Check sheet for the modelled part. Datum: model origin and axes. Units: mm. Face numbers are marked on the shaded views. A direction names the side the tool comes from. Give positions to 0.01 mm unless a question says otherwise; leave off trailing zeros. Order: outer loops, then holes, each group sorted by start corner. A loop starts at its lowest first (then second) coordinate and runs counter-clockwise, first axis right, second up.
from build123d import *

# Parameters (mm, degrees)
DODANIE_WYCI_GNI_CIE1_DEPTH  = 20
ZAAWANSOWANYOTW_R1_START     = -11.5
ZAAWANSOWANYOTW_R1_OUTLINE_R = 5.5
ZAAWANSOWANYOTW_R1_DEPTH     = 23


# Read off the part's stored shape, not the designer's step: ZaawansowanyOtwór1
with BuildPart() as part:
    # Szkic1 → Dodanie-wyciągnięcie1 (new body)
    with BuildSketch(Plane(origin=(0, 0, 0), x_dir=(1, 0, 0), z_dir=(0, 1, 0))):
        with BuildLine():
            Line((12.109500403, 11.5), (39.7, 11.5))
            ThreePointArc((39.7, 11.5), (41.114213562, 10.914213562), (41.7, 9.5))
            Line((41.7, 9.5), (41.7, 4.5))
            ThreePointArc((41.7, 4.5), (41.114213562, 3.085786438), (39.7, 2.5))
            Line((39.7, 2.5), (13.774977314, 2.5))
            Line((13.774977314, 2.5), (12.939860896, 2.5))
            ThreePointArc((12.939860896, 2.5), (11.780953784, 2.869989477), (11.050830108, 3.843065693))
            ThreePointArc((11.050830108, 3.843065693), (-11.7, 0), (11.050830108, -3.843065693))
            ThreePointArc((11.050830108, -3.843065693), (11.780953784, -2.869989477), (12.939860896, -2.5))
            Line((12.939860896, -2.5), (13.774977314, -2.5))
            Line((13.774977314, -2.5), (39.7, -2.5))
            ThreePointArc((39.7, -2.5), (41.114213562, -3.085786438), (41.7, -4.5))
            Line((41.7, -4.5), (41.7, -9.5))
            ThreePointArc((41.7, -9.5), (41.114213562, -10.914213562), (39.7, -11.5))
            Line((39.7, -11.5), (12.109500403, -11.5))
            ThreePointArc((12.109500403, -11.5), (-16.7, 0), (12.109500403, 11.5))
        make_face()
    extrude(amount=DODANIE_WYCI_GNI_CIE1_DEPTH)

    # ZaawansowanyOtwór1 outline → ZaawansowanyOtwór1 (cut)
    with BuildSketch(Plane.XY.offset(ZAAWANSOWANYOTW_R1_START)):
        with Locations((31.7, 10)):
            Circle(ZAAWANSOWANYOTW_R1_OUTLINE_R)
    extrude(amount=ZAAWANSOWANYOTW_R1_DEPTH, mode=Mode.SUBTRACT)


solid = part.part
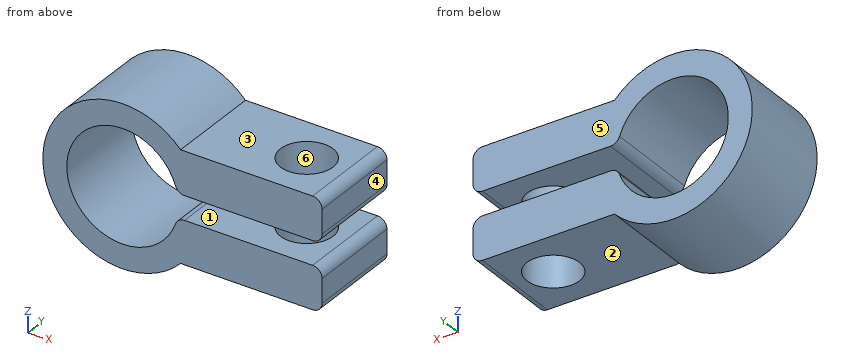
1) Depth check by flat-ended pin: pin 1 Ø4 at (x, y) = (20.5, 11) entering from +Z; pin 2 Ø10 at (x, y) = (32.5, 13) entering from -Z; pin 3 Ø6 at (y, z) = (13.5, 7) entering from -X. Enter the tip coordinate at first touch or a pass-through.
Recorded:
pin 1: stops at z = 11.5
pin 2: stops at z = -11.5
pin 3: stops at x = -16.21
2) Section check C-C, the plane z = -7. Record the cut outline in (x, y), then the cut area to 3 significant figures.
Recorded:
outline: (-15.16, 0) - (-9.37, 0) - (-9.37, 20) - (-15.16, 20) - close; (9.37, 0) - (41.7, 0) - (41.7, 20) - (9.37, 20) - close; hole circle Ø11 at (31.7, 10)
area: 667 mm2
3) Section check D-D, the plane y = 3.75. Record the cut outline in (x, z).
Recorded:
outline: (11.05, -3.84) arc R11.7 cw (long way) to (11.05, 3.84) arc R2 ccw to (12.94, 2.5) - (39.7, 2.5) arc R2 ccw to (41.7, 4.5) - (41.7, 9.5) arc R2 ccw to (39.7, 11.5) - (12.11, 11.5) arc R16.7 ccw (long way) to (12.11, -11.5) - (39.7, -11.5) arc R2 ccw to (41.7, -9.5) - (41.7, -4.5) arc R2 ccw to (39.7, -2.5) - (12.94, -2.5) arc R2 ccw to start
4) Material ranges on L1, parallel to Z at x = 14, y = 3.75; L2, parallel to Y at x = 31.7, z = 6.5; L3, parallel to X at y = 10, z = 6.75, recorded low to high.
Recorded:
L1: z = -11.5 to -2.5, 2.5 to 11.5
L2: y = 0 to 4.5, 15.5 to 20
L3: x = -15.28 to -9.56, 9.56 to 26.2, 37.2 to 41.7
5) Section check B-B, the plane y = 10. Record the cut outline in (x, z).
Recorded:
outline: (11.05, -3.84) arc R11.7 cw (long way) to (11.05, 3.84) arc R2 ccw to (12.94, 2.5) - (26.2, 2.5) - (26.2, 11.5) - (12.11, 11.5) arc R16.7 ccw (long way) to (12.11, -11.5) - (26.2, -11.5) - (26.2, -2.5) - (12.94, -2.5) arc R2 ccw to start; (37.2, -11.5) - (39.7, -11.5) arc R2 ccw to (41.7, -9.5) - (41.7, -4.5) arc R2 ccw to (39.7, -2.5) - (37.2, -2.5) - close; (37.2, 2.5) - (39.7, 2.5) arc R2 ccw to (41.7, 4.5) - (41.7, 9.5) arc R2 ccw to (39.7, 11.5) - (37.2, 11.5) - close
6) Draft check along X on the marked faces 4, 5 and 6. Enter one of: +X half, -X half, draft (parallel to the pull), parting line (faces both ways), or undercut.
Recorded:
face 4: +X half
face 5: draft
face 6: undercut
7) Section check A-A, the plane x = 0. Record the cut outline in (y, z).
Recorded:
outline: (0, -16.7) - (20, -16.7) - (20, -11.7) - (0, -11.7) - close; (0, 11.7) - (20, 11.7) - (20, 16.7) - (0, 16.7) - close
8) Set-up check for the marked faces 1, 2 and 3: record each of +Z, -Z, +X, -X, +Y, -Y from which the full face is reachable in a straight line by a thin tool's end or side.
Recorded:
face 1: +X, +Y, -Y
face 2: -Z, +X, +Y, -Y
face 3: +Z, +X, +Y, -Y
